from build123d import *

# Parameters (mm, degrees)
BOSS_EXTRUDE1_DEPTH    = 7.5
BOSS_EXTRUDE1_2_DEPTH  = 7.5
BOSS_EXTRUDE1_3_DEPTH  = 7.5
BOSS_EXTRUDE1_4_DEPTH  = 7.5
BOSS_EXTRUDE1_5_DEPTH  = 7.5
BOSS_EXTRUDE1_6_DEPTH  = 7.5
BOSS_EXTRUDE1_7_DEPTH  = 7.5
BOSS_EXTRUDE1_8_DEPTH  = 7.5
BOSS_EXTRUDE1_9_DEPTH  = 7.5
BOSS_EXTRUDE1_10_DEPTH = 7.5
BOSS_EXTRUDE1_11_DEPTH = 7.5
BOSS_EXTRUDE1_12_DEPTH = 7.5
SKETCH1_3_R            = 27
SKETCH1_3_R_2          = 25
BOSS_EXTRUDE2_DEPTH    = 10
SKETCH1_4_R            = 8.5
SKETCH1_4_R_2          = 7.5
BOSS_EXTRUDE3_DEPTH    = 7.5
SKETCH1_5_R            = 35
SKETCH1_5_R_2          = 27
BOSS_EXTRUDE4_DEPTH    = 10
SKETCH1_6_R            = 7.5
SKETCH1_6_R_2          = 2.5
BOSS_EXTRUDE5_DEPTH    = 7.5


with BuildPart() as part:
    # Sketch1 → Boss-Extrude1 (new, symmetric)
    with BuildSketch(Plane.XY):
        with BuildLine():
            Line((-25, 0), (-8.5, 0))
            ThreePointArc((-8.5, 0), (-8.43117662, 1.079472466), (-8.225820987, 2.141464239))
            Line((-8.225820987, 2.141464239), (-24.908113757, 2.141464239))
            ThreePointArc((-24.908113757, 2.141464239), (-24.977017876, 1.071717333), (-25, 0))
        make_face()
    extrude(amount=BOSS_EXTRUDE1_DEPTH, both=True)



with BuildPart() as body_2:
    # Sketch1 → Boss-Extrude1 2 (new, symmetric)
    with BuildSketch(Plane.XY):
        with BuildLine():
            ThreePointArc((-7.361215932, -4.25), (-7.84134937, -3.280737732), (-8.194502061, -2.258348061))
            Line((-8.194502061, -2.258348061), (-22.641791393, -10.599494446))
            ThreePointArc((-22.641791393, -10.599494446), (-22.166590658, -11.560374502), (-21.650635095, -12.5))
            Line((-21.650635095, -12.5), (-7.361215932, -4.25))
        make_face()
    extrude(amount=BOSS_EXTRUDE1_2_DEPTH, both=True)


with BuildPart() as body_3:
    # Sketch1 → Boss-Extrude1 3 (new, symmetric)
    with BuildSketch(Plane.XY):
        with BuildLine():
            Line((-21.650635095, 12.5), (-7.361215932, 4.25))
            ThreePointArc((-7.361215932, 4.25), (-6.761876904, 5.150438888), (-6.053037822, 5.967472926))
            Line((-6.053037822, 5.967472926), (-20.500327154, 14.308619311))
            ThreePointArc((-20.500327154, 14.308619311), (-21.094873324, 13.416643374), (-21.650635095, 12.5))
        make_face()
    extrude(amount=BOSS_EXTRUDE1_3_DEPTH, both=True)


with BuildPart() as body_4:
    # Sketch1 → Boss-Extrude1 4 (new, symmetric)
    with BuildSketch(Plane.XY):
        with BuildLine():
            ThreePointArc((-4.25, -7.361215932), (-5.150438888, -6.761876904), (-5.967472926, -6.053037822))
            Line((-5.967472926, -6.053037822), (-14.308619311, -20.500327154))
            ThreePointArc((-14.308619311, -20.500327154), (-13.416643374, -21.094873324), (-12.5, -21.650635095))
            Line((-12.5, -21.650635095), (-4.25, -7.361215932))
        make_face()
    extrude(amount=BOSS_EXTRUDE1_4_DEPTH, both=True)


with BuildPart() as body_5:
    # Sketch1 → Boss-Extrude1 5 (new, symmetric)
    with BuildSketch(Plane.XY):
        with BuildLine():
            Line((-12.5, 21.650635095), (-4.25, 7.361215932))
            ThreePointArc((-4.25, 7.361215932), (-3.280737732, 7.84134937), (-2.258348061, 8.194502061))
            Line((-2.258348061, 8.194502061), (-10.599494446, 22.641791393))
            ThreePointArc((-10.599494446, 22.641791393), (-11.560374502, 22.166590658), (-12.5, 21.650635095))
        make_face()
    extrude(amount=BOSS_EXTRUDE1_5_DEPTH, both=True)


with BuildPart() as body_6:
    # Sketch1 → Boss-Extrude1 6 (new, symmetric)
    with BuildSketch(Plane.XY):
        with BuildLine():
            ThreePointArc((0, -8.5), (-1.079472466, -8.43117662), (-2.141464239, -8.225820987))
            Line((-2.141464239, -8.225820987), (-2.141464239, -24.908113757))
            ThreePointArc((-2.141464239, -24.908113757), (-1.071717333, -24.977017876), (0, -25))
            Line((0, -25), (0, -8.5))
        make_face()
    extrude(amount=BOSS_EXTRUDE1_6_DEPTH, both=True)


with BuildPart() as body_7:
    # Sketch1 → Boss-Extrude1 7 (new, symmetric)
    with BuildSketch(Plane.XY):
        with BuildLine():
            Line((0, 25), (0, 8.5))
            ThreePointArc((0, 8.5), (1.079472466, 8.43117662), (2.141464239, 8.225820987))
            Line((2.141464239, 8.225820987), (2.141464239, 24.908113757))
            ThreePointArc((2.141464239, 24.908113757), (1.071717333, 24.977017876), (0, 25))
        make_face()
    extrude(amount=BOSS_EXTRUDE1_7_DEPTH, both=True)


with BuildPart() as body_8:
    # Sketch1 → Boss-Extrude1 8 (new, symmetric)
    with BuildSketch(Plane.XY):
        with BuildLine():
            ThreePointArc((4.25, -7.361215932), (3.280737732, -7.84134937), (2.258348061, -8.194502061))
            Line((2.258348061, -8.194502061), (10.599494446, -22.641791393))
            ThreePointArc((10.599494446, -22.641791393), (11.560374502, -22.166590658), (12.5, -21.650635095))
            Line((12.5, -21.650635095), (4.25, -7.361215932))
        make_face()
    extrude(amount=BOSS_EXTRUDE1_8_DEPTH, both=True)


with BuildPart() as body_9:
    # Sketch1 → Boss-Extrude1 9 (new, symmetric)
    with BuildSketch(Plane.XY):
        with BuildLine():
            Line((12.5, 21.650635095), (4.25, 7.361215932))
            ThreePointArc((4.25, 7.361215932), (5.150438888, 6.761876904), (5.967472926, 6.053037822))
            Line((5.967472926, 6.053037822), (14.308619311, 20.500327154))
            ThreePointArc((14.308619311, 20.500327154), (13.416643374, 21.094873324), (12.5, 21.650635095))
        make_face()
    extrude(amount=BOSS_EXTRUDE1_9_DEPTH, both=True)


with BuildPart() as body_10:
    # Sketch1 → Boss-Extrude1 10 (new, symmetric)
    with BuildSketch(Plane.XY):
        with BuildLine():
            ThreePointArc((7.361215932, -4.25), (6.761876904, -5.150438888), (6.053037822, -5.967472926))
            Line((6.053037822, -5.967472926), (20.500327154, -14.308619311))
            ThreePointArc((20.500327154, -14.308619311), (21.094873324, -13.416643374), (21.650635095, -12.5))
            Line((21.650635095, -12.5), (7.361215932, -4.25))
        make_face()
    extrude(amount=BOSS_EXTRUDE1_10_DEPTH, both=True)


with BuildPart() as body_11:
    # Sketch1 → Boss-Extrude1 11 (new, symmetric)
    with BuildSketch(Plane.XY):
        with BuildLine():
            Line((21.650635095, 12.5), (7.361215932, 4.25))
            ThreePointArc((7.361215932, 4.25), (7.84134937, 3.280737732), (8.194502061, 2.258348061))
            Line((8.194502061, 2.258348061), (22.641791393, 10.599494446))
            ThreePointArc((22.641791393, 10.599494446), (22.166590658, 11.560374502), (21.650635095, 12.5))
        make_face()
    extrude(amount=BOSS_EXTRUDE1_11_DEPTH, both=True)


with BuildPart() as body_12:
    # Sketch1 → Boss-Extrude1 12 (new, symmetric)
    with BuildSketch(Plane.XY):
        with BuildLine():
            ThreePointArc((8.5, 0), (8.43117662, -1.079472466), (8.225820987, -2.141464239))
            Line((8.225820987, -2.141464239), (24.908113757, -2.141464239))
            ThreePointArc((24.908113757, -2.141464239), (24.977017876, -1.071717333), (25, 0))
            Line((25, 0), (8.5, 0))
        make_face()
    extrude(amount=BOSS_EXTRUDE1_12_DEPTH, both=True)


with BuildPart() as part_1:
    add(part.part)

    add(body_2.part)  # Boss-Extrude2 merges body 2

    add(body_3.part)  # Boss-Extrude2 merges body 3

    add(body_4.part)  # Boss-Extrude2 merges body 4

    add(body_5.part)  # Boss-Extrude2 merges body 5

    add(body_6.part)  # Boss-Extrude2 merges body 6

    add(body_7.part)  # Boss-Extrude2 merges body 7

    add(body_8.part)  # Boss-Extrude2 merges body 8

    add(body_9.part)  # Boss-Extrude2 merges body 9

    add(body_10.part)  # Boss-Extrude2 merges body 10

    add(body_11.part)  # Boss-Extrude2 merges body 11

    add(body_12.part)  # Boss-Extrude2 merges body 12
    # Sketch1_3 → Boss-Extrude2 (add, symmetric)
    with BuildSketch(Plane.XY):
        Circle(SKETCH1_3_R)
        Circle(SKETCH1_3_R_2, mode=Mode.SUBTRACT)
    extrude(amount=BOSS_EXTRUDE2_DEPTH, both=True)

    # Sketch1_4 → Boss-Extrude3 (add, symmetric)
    with BuildSketch(Plane.XY):
        Circle(SKETCH1_4_R)
        Circle(SKETCH1_4_R_2, mode=Mode.SUBTRACT)
    extrude(amount=BOSS_EXTRUDE3_DEPTH, both=True)

    # Sketch1_5 → Boss-Extrude4 (add, symmetric)
    with BuildSketch(Plane.XY):
        Circle(SKETCH1_5_R)
        Circle(SKETCH1_5_R_2, mode=Mode.SUBTRACT)
    extrude(amount=BOSS_EXTRUDE4_DEPTH, both=True)

    # Sketch1_6 → Boss-Extrude5 (add)
    with BuildSketch(Plane.XY):
        Circle(SKETCH1_6_R)
        Circle(SKETCH1_6_R_2, mode=Mode.SUBTRACT)
    extrude(amount=BOSS_EXTRUDE5_DEPTH)


solid = part_1.part
Work out the finished part from the listing and answer in its coordinate system (mm). A direction names the side the tool comes from. Coordinates: 2 decimals unless noted, no trailing zeros. Loops run counter-clockwise (first coordinate to the right, second up) from the corner with the lowest first, then second, coordinate; pieces in that order, holes last. Notation, with made-up numbers: M 89.25,28 L 134.25,28 A27 ccw 134.25,67 Z; hole C 30,67.25 d2. An arc over 180 degrees is marked long. Answer in a Markdown table with one row per item. Add a question column.
1. The mould has two halves that part along X. Classify faces 3 (the flat face through (-6.37, 15.32, 0.11)), 4 (the cylindrical face through (-0.54, -2.44, 3.7)): pulls with the +X half, pulls with the -X half, needs draft (parallel to the pull), parting line crosses it, or undercut.
2. Find section C-C, the plane x = 26. Write down the section's boundary in (y, z), then the cut area to 3 significant figures.
3. Find section B-B, the plane y = 27.5. Write down the section's boundary in (x, z), then the cut area to 3 significant figures.
4. Flat-ended cylindrical pins translate along their axes: P1, Ø6.5, axis at x = 0, y = 0, coming from the -Z side; P2, Ø7.5, axis at x = -16.5, z = -0.5, coming from the -Y side; P3, Ø12, axis at y = 19.5, z = 3, coming from the -X side. Find the tip coordinate at first contact, or state that the pin passes through.
5. Consider L1, parallel to X at y = -19.5, z = 4.5; L2, parallel to X at y = -1, z = 5.75; L3, parallel to X at y = 22, z = 0. Determine where each line is inside the solid, lowest interval first.
6. A tool of negligible diameter and unlimited length cuts with its end or side. For faces 1 (the cylindrical face through (5.19, -6.73, 0.11)), 2 (the flat face through (-2, 2, 0)), from which of +Z, -Z, +X, -X, +Y, -Y can it reach the whole face along a straight path? Write none if from no direction.
7. Find section A-A, the plane z = 5.25. State how many separate pieces and enclosed holes the cut face has, then the cut area to 3 significant figures.
Reported:
| question | item | result |
|---|---|---|
| 1 | face 3 | undercut |
| 1 | face 4 | undercut |
| 2 | outline | M -23.43,-10 L 23.43,-10 L 23.43,10 L -23.43,10 Z |
| 2 | area | 937 mm^2 |
| 3 | outline | M -21.65,-10 L 21.65,-10 L 21.65,10 L -21.65,10 Z |
| 3 | area | 866 mm^2 |
| 4 | P1 | stops at z = 0 |
| 4 | P2 | stops at y = -32.6 |
| 4 | P3 | stops at x = -32.29 |
| 5 | L1 | x = -29.06 to -15.64, -13.73 to -11.26, -2.14 to 0, 8.79 to 11.26, 15.64 to 29.06 |
| 5 | L2 | x = -34.99 to -24.98, -8.44 to -2.29, 2.29 to 34.99 |
| 5 | L3 | x = -27.22 to -10.23, 0 to 2.14, 11.87 to 27.22 |
| 6 | face 1 | +Z, -Z |
| 6 | face 2 | -Z |
| 7 | separate pieces | 1 |
| 7 | enclosed holes | 13 |
| 7 | area | 2,520 mm^2 |
